Source: CAD feature listing. Evaluate the final solid. Frame: model axes, mm. A direction names the side the tool comes from. Round coordinates to 2 decimals unless told otherwise and drop trailing zeros. Order: outer loops, then holes, each group sorted by start corner. A loop starts at its lowest first (then second) coordinate and runs counter-clockwise, first axis right, second up. Notation, with made-up numbers: (56.5, 21.5) - (112.5, 21.5) arc R26 cw to (112.5, 46.5) - close; hole circle Ø3 at (60.5, -16). An arc over 180 degrees is marked (long way). Put each result on its own line as item: value. Start each with the question number.
1) Section B-B on x = 0. Output: boundary loops of the cut face in (y, z), then the cut area to 3 significant figures.
2) Access query for faces 4 (the face through (13.687, -7.832, 2.425)), 5 (the face through (0, 0, 0)). Directions: +Z, -Z, +X, -X, +Y, -Y. A direction counts if a zero-diameter tool reaches every point of the face in a straight line with its end or side. Return the directions, or none.
3) Mould query, pull axis Z, two halves, no side actions, for faces 1 (the face through (0, -13, -13.234)), 2 (the face through (14, -6, -10)), 3 (the face through (0, -25.4, -3)). Classes: +Z half, -Z half, draft (parallel to the pull), parting line (faces both ways), or undercut.
4) Section A-A on z = -10. State how many separate pieces and enclosed holes the cut face has, then the cut area to 3 significant figures.
5) Line query: probe 1 along Y at (x, z) = (10.5, 12); probe 2 along X at (y, z) = (-1.25, 3.5); probe 3 along X at (y, z) = (-23.5, -8). Output: solid intervals per line, ascending. Write a range as [from, to].
```python
from build123d import *

# Parameters (mm, degrees)
F0_W     = 29.1386954486
F0_H     = 26.4676492661
F1_DEPTH = 25.4
F2_R     = 2.7472233706
F3_DEPTH = 5.08
F3_TAPER = -30
F4_R     = 2.54
F5_DEPTH = 5.08
F5_TAPER = -30
F6_R     = 2.54
F7_DEPTH = 5.08
F7_TAPER = -30


with BuildPart() as f1:
    # F0 (on Front) → F1 (new body)
    with BuildSketch(Plane.XZ):
        Rectangle(F0_W, F0_H)
    extrude(amount=F1_DEPTH)

    # F2 (on face) → F3 (cut)
    with BuildSketch(Plane.XY.offset(13.2338246331)):
        with Locations((0, -12.2625352815)):
            Circle(F2_R)
    extrude(amount=-F3_DEPTH, taper=F3_TAPER, mode=Mode.SUBTRACT)

    # F4 (on face) → F5 (cut)
    with BuildSketch(Plane.XZ.offset(25.4)):
        with Locations((8.7416088209, -8.1345522776)):
            Circle(F4_R)
        Circle(F4_R)
        with Locations((-9.4700763002, 9.5914872363)):
            Circle(F4_R)
    extrude(amount=-F5_DEPTH, taper=F5_TAPER, mode=Mode.SUBTRACT)

    # F6 (on face) → F7 (cut)
    with BuildSketch(Plane.YZ.offset(14.5693477243)):
        with Locations((-20.3970875591, 8.1345522776)):
            Circle(F6_R)
        with Locations((-19.911441952, 0.1214112272)):
            Circle(F6_R)
        with Locations((-20.8827313036, -7.6489071362)):
            Circle(F6_R)
        with Locations((-5.5849160999, -7.1632624604)):
            Circle(F6_R)
        with Locations((-5.5849160999, 0.3642337106)):
            Circle(F6_R)
        with Locations((-5.342093762, 7.8917304054)):
            Circle(F6_R)
    extrude(amount=-F7_DEPTH, taper=F7_TAPER, mode=Mode.SUBTRACT)


solid = f1.part
```
Answer sheet:
1. outline: (-25.4, -13.23) - (0, -13.23) - (0, 13.23) - (-9.52, 13.23) - (-6.58, 8.15) - (-17.94, 8.15) - (-15.01, 13.23) - (-25.4, 13.23) - (-25.4, 2.54) - (-20.32, 5.47) - (-20.32, -5.47) - (-25.4, -2.54) - close
1. area: 589 mm^2
2. face 4: none
2. face 5: +Z, -Z, +X, -X, +Y
3. face 1: -Z half
3. face 2: undercut
3. face 3: draft
4. separate pieces: 2
4. enclosed holes: 1
4. area: 660 mm^2
5. probe 1: [-25.4, -23.39], [-17.4, -7.99], [-2.69, 0]
5. probe 2: [-14.57, 9.49], [9.7, 14.57]
5. probe 3: [-14.57, 5.11], [14.39, 14.57]
